For this review, take the finished solid that the model builds, in its own axes (mm). Round coordinates to 2 decimals unless told otherwise and drop trailing zeros. Write each loop counter-clockwise with the first axis right and the second up, starting at its lowest first coordinate (ties: lowest second). Pieces come first, ordered by that corner, then holes. Notation, with made-up numbers: (-37.75, -16.5) -> (-1.75, -16.5) arc R9 cw to (-1.75, -3.5) -> close; hole circle Ø2 at (40.25, -23). An arc over 180 degrees is marked (long way). Answer in a Markdown table with one row per item.
Autodesk Inventor part; units mm, degrees
ref_plane "YZ Plane" through (0, 0, 0) normal (1, 0, 0) x (0, 1, 0)
ref_plane "XZ Plane" through (0, 0, 0) normal (0, 1, 0) x (-1, 0, 0)
ref_plane "XY Plane" through (0, 0, 0) normal (0, 0, 1) x (1, 0, 0)
sketch "スケッチ1" plane through (0, 0, 0) normal (0, 1, 0) x (-1, 0, 0)
  line L0 (-550, 330) -> (550, 330)
  line L1 (550, 330) -> (550, -330)
  line L2 (550, -330) -> (-550, -330)
  line L3 (-550, -330) -> (-550, 330)
  line L4 (-550, 330) -> (550, -330) construction
  line L5 (550, 330) -> (-550, -330) construction
  line L6 (427, 75) -> (349, 75)
  line L7 (334, 60) -> (334, -60)
  line L8 (349, -75) -> (427, -75)
  line L9 (442, -60) -> (442, 60)
  line L10 (442, 75) -> (334, -75) construction
  line L11 (334, 75) -> (442, -75) construction
  arc A0 (442, 60) -> (427, 75) centre (427, 60) ccw
  arc A1 (349, 75) -> (334, 60) centre (349, 60) ccw
  arc A2 (427, -75) -> (442, -60) centre (427, -60) ccw
  arc A3 (334, -60) -> (349, -75) centre (349, -60) ccw
  circle A4 centre (-530, 310) radius 5
  circle A5 centre (-530, -310) radius 5
  circle A6 centre (-530, 0) radius 5
  circle A7 centre (-530, 155) radius 5
  circle A8 centre (-530, -155) radius 5
  line L12 (0, -462) -> (0, 462)
  circle A9 centre (530, 310) radius 5
  circle A10 centre (530, -310) radius 5
  circle A11 centre (530, 0) radius 5
  circle A12 centre (530, 155) radius 5
  circle A13 centre (530, -155) radius 5
  circle A14 centre (318, 310) radius 5
  circle A15 centre (106, 310) radius 5
  circle A16 centre (-106, 310) radius 5
  circle A17 centre (-318, 310) radius 5
  line L13 (770, 0) -> (-770, 0)
  circle A18 centre (318, -310) radius 5
  circle A19 centre (106, -310) radius 5
  circle A20 centre (-106, -310) radius 5
  circle A21 centre (-318, -310) radius 5
  point P0 (0, 0)
  point P1 (388, 0)
  point P2 (0, -250)
  point P3 (0, -125)
  point P4 (0, 125)
  point P5 (0, 250)
  dimension "d0" = 1100
  dimension "d1" = 660
  dimension "d2" = 108
  dimension "d3" = 108
  dimension "d4" = 150
  dimension "d5" = 255
  dimension "d6" = 15
  dimension "d7" = 15
  dimension "d8" = 10
  dimension "d9" = 20
  dimension "d10" = 20
  dimension "d11" = 10
  dimension "d12" = 20
  dimension "d13" = 20
  dimension "d14" = 10
  dimension "d15" = 10
  dimension "d16" = 155
  dimension "d17" = 10
  dimension "d18" = 155
  dimension "d19" = 20
  dimension "d20" = 20
  dimension "d21" = 20
  dimension "d24" = 212
  dimension "d185" = 80
  dimension "d186" = 205
  dimension "d187" = 80
  dimension "d188" = 205
extrude "押し出し1" add sketch "スケッチ1" along normal blind 20 contours L0 L12 L13 A6 L3 | L0 L1 L13 A11 L9 A0 L6 A1 L7 L12 | L13 A6 L12 L2 L3 | L13 L7 A3 L8 A2 L9 A11 L1 L2 L12
extrude "押し出し2" add sketch "スケッチ1" along normal blind 20 contours A9 | A14 | A15 | A16 | A17
extrude "押し出し3" cut sketch "スケッチ1" along normal blind 20 contours L13 A6 | A6 L13 | L13 A11 | A11 L13 | A4 | A5 | A7 | A8 | A10 | A12 | A13 | A17 | A18 | A19 | A20 | A21
extrude "押し出し4" add sketch "スケッチ1" along normal blind 20 contours L13 A11 | A11 L13 | A10 | A12 | A13 | A18 | A19
extrude "押し出し5" add sketch "スケッチ1" along normal blind 20 contours L0 L12 L13 A6 L3 | L0 L1 L13 A11 L9 A0 L6 A1 L7 L12 | L13 A6 L12 L2 L3 | L13 L7 A3 L8 A2 L9 A11 L1 L2 L12 | L13 A6 | A6 L13 | A5 | A8 | A20 | A21
extrude "押し出し6" add sketch "スケッチ1" along normal blind 20 contours L0 L12 L13 A6 L3 | L0 L1 L13 A11 L9 A0 L6 A1 L7 L12 | L13 A6 L12 L2 L3 | L13 L7 A3 L8 A2 L9 A11 L1 L2 L12 | A4 | A7 | A17
hole "穴1" at (530, 0, 310) direction (0, 1, 0) diameter 8 depth 20 counterbore diameter 12 counterbore depth 6
hole "穴2" at (318, 0, 310) direction (0, 1, 0) diameter 8 depth 20 counterbore diameter 12 counterbore depth 6
hole "穴3" at (106, 0, 310) direction (0, 1, 0) diameter 8 depth 20 counterbore diameter 12 counterbore depth 6
hole "穴4" at (-106, 0, 310) direction (0, 1, 0) diameter 8 depth 20 counterbore diameter 12 counterbore depth 6
hole "穴5" at (-318, 0, 310) direction (0, 1, 0) diameter 8 depth 20 counterbore diameter 12 counterbore depth 6
hole "穴6" at (-530, 0, 310) direction (0, 1, 0) diameter 8 depth 20 counterbore diameter 12 counterbore depth 6
hole "穴7" at (-530, 0, 155) direction (0, 1, 0) diameter 8 depth 20 counterbore diameter 12 counterbore depth 6
hole "穴8" at (-530, 0, 0) direction (0, 1, 0) diameter 8 depth 20 counterbore diameter 12 counterbore depth 6
hole "穴9" at (-530, 0, -155) direction (0, 1, 0) diameter 8 depth 20 counterbore diameter 12 counterbore depth 6
hole "穴10" at (-530, 0, -310) direction (0, 1, 0) diameter 8 depth 20 counterbore diameter 12 counterbore depth 6
hole "穴11" at (-318, 0, -310) direction (0, 1, 0) diameter 8 depth 20 counterbore diameter 12 counterbore depth 6
hole "穴12" at (-106, 0, -310) direction (0, 1, 0) diameter 8 depth 20 counterbore diameter 12 counterbore depth 6
hole "穴13" at (106, 0, -310) direction (0, 1, 0) diameter 8 depth 20 counterbore diameter 12 counterbore depth 6
hole "穴14" at (318, 0, -310) direction (0, 1, 0) diameter 8 depth 20 counterbore diameter 12 counterbore depth 6
hole "穴15" at (530, 0, -310) direction (0, 1, 0) diameter 8 depth 20 counterbore diameter 12 counterbore depth 6
hole "穴16" at (530, 0, -155) direction (0, 1, 0) diameter 8 depth 20 counterbore diameter 12 counterbore depth 6
hole "穴17" at (530, 0, 0) direction (0, 1, 0) diameter 8 depth 20 counterbore diameter 12 counterbore depth 6
hole "穴18" at (530, 0, 155) direction (0, 1, 0) diameter 8 depth 20 counterbore diameter 12 counterbore depth 6
fillet "フィレット1" radius 2 4 edges at (550, 10, -330) (-550, 10, -330) (-550, 10, 330) (550, 10, 330)
hole "穴19" at (0, 0, -250) at (0, 0, -125) at (0, 0, 125) at (0, 0, 250) direction (0, 1, 0) diameter 8 depth 20 counterbore diameter 12 counterbore depth 6
properties part number "board" material "ステンレス鋼"
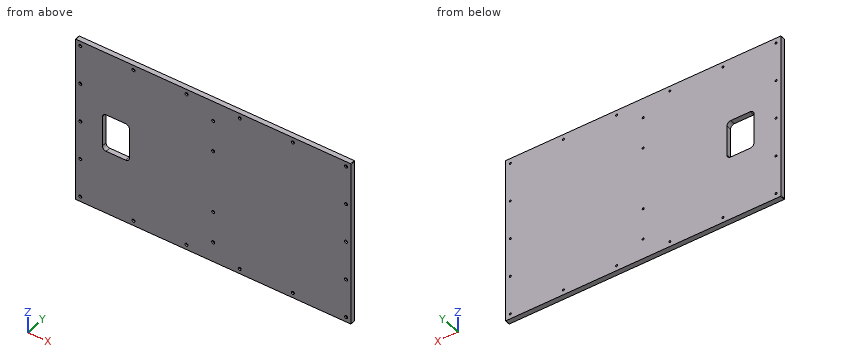
1) Consider section B-B on y = 16.5. State how many separate pieces and enclosed holes the cut face has, then the cut area to 3 significant figures.
Solved:
| item | result |
|---|---|
| separate pieces | 1 |
| enclosed holes | 23 |
| area | 709,000 mm² |
2) For line 1 (X direction, y = 14, z = 154); line 2 (X direction, y = 16, z = 0); line 3 (Z direction, x = 0, y = 1.5), list the stretches that pass through material, from the lowest coordinate up. Write a range as [from, to].
Solved:
| item | result |
|---|---|
| line 1 | [-550, -533.87], [-526.13, 526.13], [533.87, 550] |
| line 2 | [-550, -534], [-526, -442], [-334, 526], [534, 550] |
| line 3 | [-330, -256], [-244, -131], [-119, 119], [131, 244], [256, 330] |
3) Consider section A-A on z = 27. State the section outline as (x, y) points, then the cut area to 3 significant figures.
Solved:
| item | result |
|---|---|
| outline | (-550, 0) -> (-442, 0) -> (-442, 20) -> (-550, 20) -> close; (-334, 0) -> (550, 0) -> (550, 20) -> (-334, 20) -> close |
| area | 19,800 mm² |
4) Clearance check with flat-ended pins moving along their axes: pin 1 Ø9 at (x, z) = (106, 310) entering from +Y; pin 2 Ø11 at (x, z) = (-530, -155) entering from -Y; pin 3 Ø3.5 at (x, z) = (-317.5, -310) entering from -Y. State where each tip first meets the part, or that it passes through.
Solved:
| item | result |
|---|---|
| pin 1 | y = 20 |
| pin 2 | y = 6 |
| pin 3 | through |
